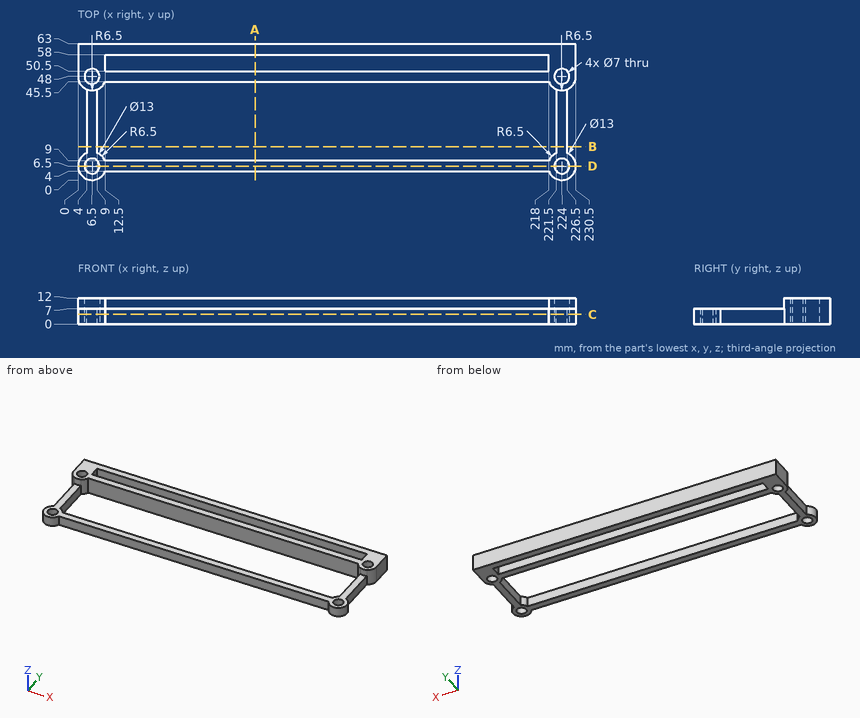
For this review, use the dimensioned drawing (mm, ordinates from the lowest corner) and the shaded views. Round coordinates to 2 decimals unless told otherwise and drop trailing zeros. Write each loop counter-clockwise with the first axis right and the second up, starting at its lowest first coordinate (ties: lowest second). Pieces come first, ordered by that corner, then holes. Notation, with made-up numbers: (16.5, 74.25) - (33.5, 74.25) arc R18 ccw to (33.5, 100.25) - close; hole circle Ø10 at (59, 57). An arc over 180 degrees is marked (long way). One line per item, written item: value. Start each with the question number.
1. Consider section A-A on x = 82. Write out the cut boundary in (y, z), and give its area (3 significant figures).
2. Consider section C-C on z = 4.5. Write out the cut boundary in (x, y), and give its area (4 significant figures).
3. Consider section B-B on y = 15.5. Write out the cut boundary in (x, z), and give its area (3 significant figures).
4. Clearance check with flat-ended pins moving along their axes: P1, Ø11, axis at x = 224, y = 48, coming from the +Z side; P2, Ø3.5, axis at y = 32.5, z = 3, coming from the +X side; P3, Ø5.5, axis at x = 6.5, y = 6.5, coming from the -Z side; P4, Ø5.5, axis at x = 76.5, z = 4, coming from the -Y side. State where each tip first meets the part, or that it passes through.
5. To check wall thickness, follow L1, parallel to X at y = 48, z = 5.25; L2, parallel to Y at x = 176.5, z = 2.5; L3, parallel to Y at x = 6.5, z = 4.25. State the ranges of each line that lie inside material, in increasing order. Write a range as from..to.
6. Consider section D-D on y = 6.5. Write out the cut boundary in (x, z), and give its area (3 significant figures).
Checks:
1. outline: (4, 0) - (9, 0) - (9, 7) - (4, 7) - close; (45.5, 0) - (50.5, 0) - (50.5, 12) - (45.5, 12) - close; (58, 0) - (63, 0) - (63, 12) - (58, 12) - close
1. area: 155 mm^2
2. outline: (0, 48) arc R6.5 ccw to (4, 42) - (4, 12.5) arc R6.5 ccw (long way) to (12.5, 4) - (218, 4) arc R6.5 ccw (long way) to (226.5, 12.5) - (226.5, 42) arc R6.5 ccw to (230.5, 48) - (230.5, 63) - (0, 63) - close; hole circle Ø7 at (6.5, 6.5); hole circle Ø7 at (6.5, 48); hole (9, 12.5) arc R6.5 cw to (12.5, 9) - (218, 9) arc R6.5 cw to (221.5, 12.5) - (221.5, 42) arc R6.5 cw to (218, 45.5) - (12.5, 45.5) arc R6.5 cw to (9, 42) - close; hole (12.5, 50.5) - (218, 50.5) - (218, 58) - (12.5, 58) - close; hole circle Ø7 at (224, 6.5); hole circle Ø7 at (224, 48)
2. area: 3,985 mm^2
3. outline: (4, 0) - (9, 0) - (9, 7) - (4, 7) - close; (221.5, 0) - (226.5, 0) - (226.5, 7) - (221.5, 7) - close
3. area: 70.0 mm^2
4. P1: stops at z = 12
4. P2: stops at x = 226.5
4. P3: passes through
4. P4: stops at y = 4
5. L1: x = 0..3, 10..220.5, 227.5..230.5
5. L2: y = 4..9, 45.5..50.5, 58..63
5. L3: y = 0..3, 10..44.5, 51.5..63
6. outline: (0, 0) - (3, 0) - (3, 7) - (0, 7) - close; (10, 0) - (220.5, 0) - (220.5, 7) - (10, 7) - close; (227.5, 0) - (230.5, 0) - (230.5, 7) - (227.5, 7) - close
6. area: 1,520 mm^2
